from build123d import *

# Parameters (mm, degrees)
F2_DEPTH = 63.5
F4_DEPTH = 38.1
F5_DEPTH = 76.2


with BuildPart() as f1:
    # F0 (on Front) → F1 (revolve)
    with BuildSketch(Plane.XZ):
        with BuildLine():
            Line((0, 1155.7), (63.5, 1155.7))
            Line((63.5, 1155.7), (63.5, 1993.9))
            Line((63.5, 1993.9), (55.5625, 2057.4))
            Line((55.5625, 2057.4), (55.5625, 2221.968274071))
            Line((55.5625, 2221.968274071), (108.1740037456, 2236.0654840123))
            ThreePointArc((108.1740037456, 2236.0654840123), (121.7511748434, 2245.1374597032), (127, 2260.6))
            Line((127, 2260.6), (139.7, 2260.6))
            Line((139.7, 2260.6), (139.7, 2387.6))
            Line((139.7, 2387.6), (0, 2387.6))
            Line((0, 2387.6), (0, 1155.7))
        make_face()
    revolve(axis=Axis((0, 0, 1771.65), (0, 0, -1)))



with BuildPart() as f1b:
    # F0 (on Front) → F1, piece 2 (revolve)
    with BuildSketch(Plane.XZ):
        Polygon((0, 774.7), (0, 0), (44.45, 0), (44.45, 50.8), (50.8, 69.85), (63.5, 774.7), align=None)
    revolve(axis=Axis((0, 0, 1771.65), (0, 0, -1)))


with BuildPart() as f1_1:
    add(f1.part)

    add(f1b.part)  # F2 merges F1b
    # F0 (on Front) → F2 (join, symmetric)
    with BuildSketch(Plane.XZ):
        Polygon((-63.5, 774.7), (0, 774.7), (63.5, 774.7), (63.5, 1155.7), (0, 1155.7), (-63.5, 1155.7), align=None)
    extrude(amount=F2_DEPTH, both=True)

    # F3 (on face) → F4 (cut)
    with BuildSketch(Plane.XY.offset(2387.6)):
        with BuildLine():
            ThreePointArc((43.7065244499, -62.4193857748), (67.5902254882, -35.1852443285), (76.2, 0))
            ThreePointArc((76.2, 0), (67.5902254882, 35.1852443285), (43.7065244499, 62.4193857748))
            ThreePointArc((43.7065244499, 62.4193857748), (0, 76.2), (-43.7065244499, 62.4193857748))
            ThreePointArc((-43.7065244499, 62.4193857748), (-76.2, 0), (-43.7065244499, -62.4193857748))
            ThreePointArc((-43.7065244499, -62.4193857748), (0, -76.2), (43.7065244499, -62.4193857748))
        make_face()
    extrude(amount=-F4_DEPTH, mode=Mode.SUBTRACT)

    # F3 (on face) → F5 (cut)
    with BuildSketch(Plane.XY.offset(2387.6)):
        with BuildLine():
            ThreePointArc((-43.7065244499, -62.4193857748), (-76.2, 0), (-43.7065244499, 62.4193857748))
            Line((-43.7065244499, 62.4193857748), (-80.1286281582, 114.4355405872))
            ThreePointArc((-80.1286281582, 114.4355405872), (-139.7, 0), (-80.1286281582, -114.4355405872))
            Line((-80.1286281582, -114.4355405872), (-43.7065244499, -62.4193857748))
        make_face()
        with BuildLine():
            ThreePointArc((43.7065244499, 62.4193857748), (67.5902254882, 35.1852443285), (76.2, 0))
            ThreePointArc((76.2, 0), (67.5902254882, -35.1852443285), (43.7065244499, -62.4193857748))
            Line((43.7065244499, -62.4193857748), (80.1286281582, -114.4355405872))
            ThreePointArc((80.1286281582, -114.4355405872), (123.915413395, -64.5062812689), (139.7, 0))
            ThreePointArc((139.7, 0), (123.915413395, 64.5062812689), (80.1286281582, 114.4355405872))
            Line((80.1286281582, 114.4355405872), (43.7065244499, 62.4193857748))
        make_face()
    extrude(amount=-F5_DEPTH, mode=Mode.SUBTRACT)


solid = f1_1.part
Input: part model. Units: mm. Frame: model coordinates. A direction names the side the tool comes from. Round coordinates to 2 decimals unless told otherwise and drop trailing zeros. Order: outer loops, then holes, each group sorted by start corner. A loop starts at its lowest first (then second) coordinate and runs counter-clockwise, first axis right, second up. Notation, with made-up numbers: (-4.5, 73.25) - (30.5, 73.25) arc R19 cw to (30.5, 81.25) - close; hole circle Ø5 at (3, -26.75). An arc over 180 degrees is marked (long way). Answer as a JSON object with one key per item and string values. Group by question number.
(1) Reachability of faces 1 (the face through (51, 48, 1155.7)), 2 (the face through (50, 50, 774.7)), 3 (the face through (-13.77, 61.99, 1580.67)), 4 (the face through (-0.652, -76.197, 2368.817)), 5 (the face through (-61.66, 88.06, 2350.03)) from +Z, -Z, +X, -X, +Y, -Y: full face, straight path, thin tool, end or side. Return the list, or none.
(2) Cut plane A-A (z = 806). Return loops of the section in (x, y), then the cut area to 3 significant figures.
(3) Draft query along Z for faces 6 (the face through (48, -51, 774.7)), 7 (the face through (-7.23, -55.09, 2140.84)), 8 (the face through (-63.5, -1, 968)). Return one class per face: released by +Z, released by -Z, zero draft, split by the parting line, or undercut.
(4) Material intervals for probe 1 along X at (y, z) = (-27, 117.5); probe 2 along X at (y, z) = (45, 1945.5); probe 3 along Z at (x, y) = (-44, 47), sorted ascending. Write a range as from..to.
(5) Cut plane B-B (z = 1754). Return loops of the section in (x, y).
(6) Pin query (flat end, axial travel): P1, Ø2, axis at x = 88.5, y = 13.5, coming from the -Z side; P2, Ø3, axis at y = 36.5, z = 1948, coming from the -X side; P3, Ø5, axis at x = 8.5, z = 341.5, coming from the -Y side. Return the tip coordinate at first contact, or that it passes through.
Here are the results:
{
 "1": {"face 1": "+X, +Y", "face 2": "-Z, +X, +Y", "face 3": "none", "face 4": "+Z", "face 5": "+Z, -X"},
 "2": {"outline": "(-63.5, -63.5) - (63.5, -63.5) - (63.5, 63.5) - (-63.5, 63.5) - close", "area": "16,100 mm^2"},
 "3": {"face 6": "released by -Z", "face 7": "undercut", "face 8": "zero draft"},
 "4": {"probe 1": "x = -44.04..44.04", "probe 2": "x = -44.8..44.8", "probe 3": "z = 774.7..1155.7, 2224.33..2349.5"},
 "5": {"outline": "circle Ø127 at (0, 0)"},
 "6": {"P1": "stops at z = 2230.8", "P2": "stops at x = -52.98", "P3": "stops at y = -55.37"}
}
